Drawing for the job (mm, zero at the part's lowest x, y, z). A direction names the side the tool comes from. Round coordinates to 2 decimals unless told otherwise and drop trailing zeros. Loops run counter-clockwise (first coordinate to the right, second up) from the corner with the lowest first, then second, coordinate; pieces in that order, holes last. Notation, with made-up numbers: (-29, -16.5) -> (-1, -16.5) arc R24 cw to (-1, 15.5) -> close; hole circle Ø7 at (41.5, 89.5). An arc over 180 degrees is marked (long way). Put each result on its own line as item: value. Start each with the question number.
Item 1: Cut at B-B, the plane x = 25.5. List the corners of the cut face in (y, z) (3 decimals).
Item 2: Cut at C-C, the plane z = 132. List the corners of the cut face in (x, y) (3 decimals).
Item 3: Pull direction Y, two halves, no side cores. Call the marked faces 3, 4 and 5: +Y half, -Y half, draft (parallel to the pull), parting line (faces both ways), or undercut.
Item 4: Flat gauge pin, fed straight in: pin 1 Ø14.5 at (y, z) = (38.1, 181.41) entering from +X. Where does the tip first touch, or does it go through?
Item 5: Drill centre lines: probe 1 along Z at (x, y) = (75, 38); probe 2 along X at (y, z) = (54, 51) (3 decimals). Where is each one in solid material? Low to high. Write a range as [from, to].
Item 6: Tool access for the marked faces 1 and 2: list every direction of +Z, -Z, +X, -X, +Y, -Y with a clear straight run to the whole face (end or side of a thin tool).
Item 7: Cut at A-A, the plane y = 38.1. Count the separate pieces of the cut face and the enclosed holes in it, plus the area to 3 significant figures.
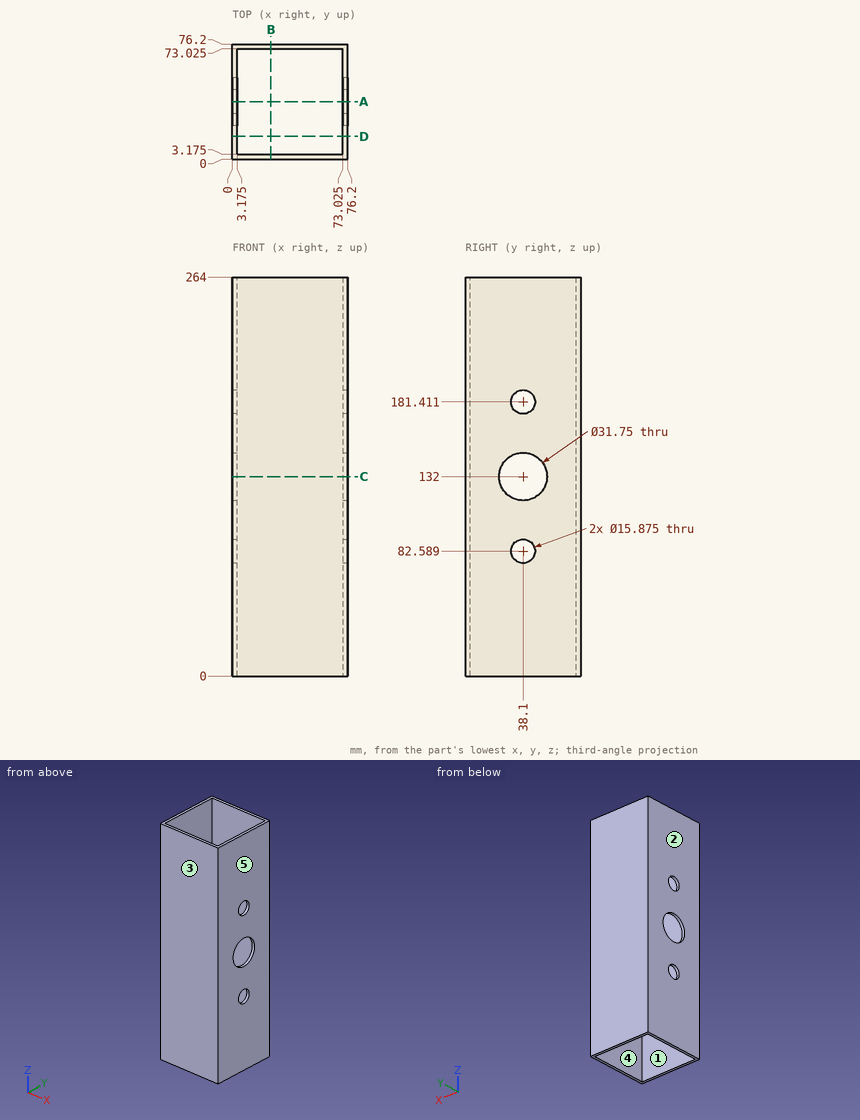
Reply:
1. outline: (0, 0) -> (3.175, 0) -> (3.175, 264) -> (0, 264) -> close; (73.025, 0) -> (76.2, 0) -> (76.2, 264) -> (73.025, 264) -> close
2. outline: (0, 0) -> (76.2, 0) -> (76.2, 22.225) -> (73.025, 22.225) -> (73.025, 3.175) -> (3.175, 3.175) -> (3.175, 22.225) -> (0, 22.225) -> close; (0, 53.975) -> (3.175, 53.975) -> (3.175, 73.025) -> (73.025, 73.025) -> (73.025, 53.975) -> (76.2, 53.975) -> (76.2, 76.2) -> (0, 76.2) -> close
3. face 3: -Y half
3. face 4: undercut
3. face 5: draft
4. pin 1: passes through
5. probe 1: z = [0, 74.65], [90.53, 116.13], [147.87, 173.47], [189.35, 264]
5. probe 2: x = [0, 3.175], [73.025, 76.2]
6. face 1: +Z, -Z
6. face 2: +Z, -Z, -X, +Y, -Y
7. separate pieces: 8
7. enclosed holes: 0
7. area: 1,270 mm^2
